Verification items for this drawing (mm, ordinates from the low corner). Round coordinates to 2 decimals unless told otherwise and drop trailing zeros. Loops run counter-clockwise (first coordinate to the right, second up) from the corner with the lowest first, then second, coordinate; pieces in that order, holes last. Notation, with made-up numbers: (54.5, -36.5) - (113.5, -36.5) arc R38 cw to (113.5, 2.5) - close; hole circle Ø8 at (69.25, 42.25). An arc over 180 degrees is marked (long way). Put each result on its own line as item: value.
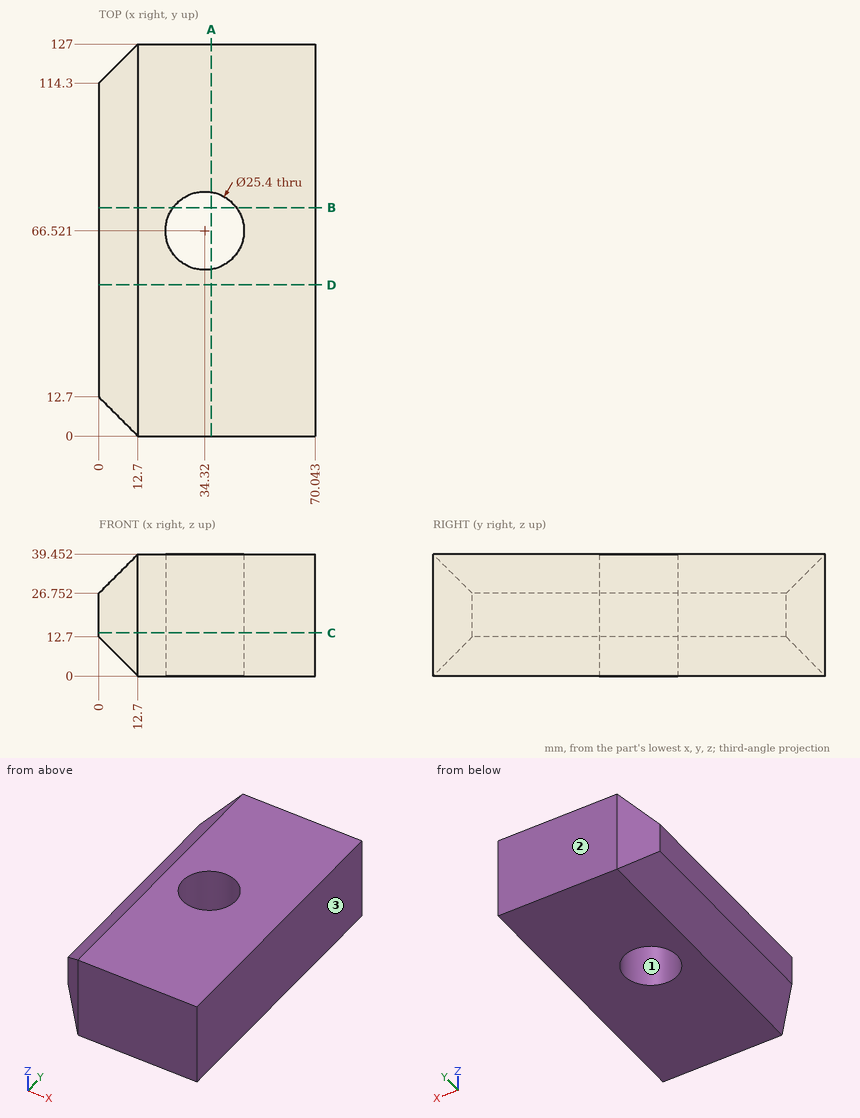
Item 1: Section check C-C on z = 14. Enter the section's corners in (x, y), then the cut area to 3 significant figures.
Filled sheet:
outline: (0, 12.7) - (12.7, 0) - (70.04, 0) - (70.04, 127) - (12.7, 127) - (0, 114.3) - close; hole circle Ø25.4 at (34.32, 66.52)
area: 8,230 mm²
Item 2: Section check B-B on y = 74. Enter the section's corners in (x, z) (1 decimal).
Filled sheet:
outline: (0, 12.7) - (12.7, 0) - (24.1, 0) - (24.1, 39.5) - (12.7, 39.5) - (0, 26.8) - close; (44.6, 0) - (70, 0) - (70, 39.5) - (44.6, 39.5) - close
Item 3: Release check for a two-part mould opening along X. For the marked faces 1, 2 and 3 record: +X half, -X half, draft (parallel to the pull), parting line (faces both ways), or undercut.
Filled sheet:
face 1: undercut
face 2: draft
face 3: +X half
Item 4: Section check A-A on x = 36.5. Enter the section's corners in (y, z), then the cut area to 3 significant figures.
Filled sheet:
outline: (0, 0) - (54.01, 0) - (54.01, 39.45) - (0, 39.45) - close; (79.03, 0) - (127, 0) - (127, 39.45) - (79.03, 39.45) - close
area: 4,020 mm²
Item 5: Go/stop test with flat-tipped pins: pin 1 (1.5 mm diameter, centred on y = 63, z = 34.5, fed in from -X); pin 2 (1.5 mm diameter, centred on y = 96, z = 8.5, fed in from -X); pin 3 (1 mm diameter, centred on x = 19, z = 5, fed in from -Y). Record where each tip stops, or that it passes through.
Filled sheet:
pin 1: x = 7
pin 2: x = 3.45
pin 3: y = 0
Item 6: Section check D-D on y = 49. Enter the section's corners in (x, z), then the cut area to 3 significant figures.
Filled sheet:
outline: (0, 12.7) - (12.7, 0) - (70.04, 0) - (70.04, 39.45) - (12.7, 39.45) - (0, 26.75) - close
area: 2,600 mm²
Item 7: Thickness scan on line 1 (Y direction, x = 30, z = 7.5); line 2 (Y direction, x = 33, z = 33); line 3 (Y direction, x = 5.5, z = 11). Record the ranges inside material, lowest first. Write a range as from..to.
Filled sheet:
line 1: 0..54.58, 78.46..127
line 2: 0..53.89, 79.15..127
line 3: 7.2..119.8
